Autodesk Inventor part; units mm, degrees
ref_plane "YZ Plane" through (0, 0, 0) normal (1, 0, 0) x (0, 1, 0)
ref_plane "XZ Plane" through (0, 0, 0) normal (0, 1, 0) x (-1, 0, 0)
ref_plane "XY Plane" through (0, 0, 0) normal (0, 0, 1) x (1, 0, 0)
sketch "Sketch1" plane through (0, 0, 0) normal (0, 0, 1) x (1, 0, 0)
  circle A0 centre (0, 0) radius 21
  circle A1 centre (16, 0) radius 2.75
  circle A2 centre (0, 16) radius 2.75
  circle A3 centre (-16, 0) radius 2.75
  circle A4 centre (0, -16) radius 2.75
  circle A5 centre (0, 0) radius 11.1
  dimension "d0" = 42
  dimension "d1" = 5.5
  dimension "d2" = 16
  dimension "d5" = 360
  dimension "d7" = 22.2
extrude "Extrusion1" add sketch "Sketch1" along normal blind 15
sketch "Sketch2" plane through (0, 0, 15) normal (0, 0, 1) x (1, 0, 0)
  circle A0 centre (0, 0) radius 19.1
  dimension "d10" = 38.2
extrude "Extrusion2" cut sketch "Sketch2" against normal blind 2.3
chamfer "Chamfer1" distance 0.5 angle 45 9 edges at (-21, 0, 0) (-21, 0, 15) (-11.1, 0, 0) (-2.75, -16, 0) (-2.75, 16, 0) (13.25, 0, 0) (-18.75, 0, 0) (-11.1, 0, 12.7) (-19.1, 0, 15)
properties part number "spacer nema23" material "PC/ABS Plastic"
The model under review builds one solid part; all positions refer to its coordinate system, in mm. A direction names the side the tool comes from. Round coordinates to 2 decimals unless told otherwise and drop trailing zeros. Loops run counter-clockwise (first coordinate to the right, second up) from the corner with the lowest first, then second, coordinate; pieces in that order, holes last. Notation, with made-up numbers: M 38.25,-10.5 L 77.25,-10.5 A23 ccw 77.25,9.5 Z; hole C 40,-37.5 d3. An arc over 180 degrees is marked long. Answer as a JSON object with one key per item and string values.
Item 1: Clearance check with flat-ended pins moving along their axes: P1, Ø4, axis at y = -13.5, z = 8, coming from the -X side; P2, Ø12, axis at x = 8.5, y = 15, coming from the -Z side; P3, Ø1.5, axis at x = 0.5, y = 11, coming from the +Z side; P4, Ø4, axis at y = -11, z = 12, coming from the -X side. State where each tip first meets the part, or that it passes through.
Check sheet entries:
{"P1": "x = -17.57", "P2": "z = 0", "P3": "z = 12.7", "P4": "x = -18.97"}
Item 2: We need section A-A, the plane y = 0. State how many separate pieces and enclosed holes the cut face has, and give its area (3 significant figures).
Check sheet entries:
{"separate pieces": "4", "enclosed holes": "0", "area": "119 mm2"}
Item 3: For line 1 along Y through (x, z) = (0, 10); line 2 along Y through (x, z) = (2, 11.25); line 3 along Y through (x, z) = (0, 13.95), list the stretches that pass through material, from the lowest coordinate up.
Check sheet entries:
{"line 1": "-21 to -18.75, -13.25 to -11.1, 11.1 to 13.25, 18.75 to 21", "line 2": "-20.9 to -17.89, -14.11 to -10.92, 10.92 to 14.11, 17.89 to 20.9", "line 3": "-21 to -19.1, 19.1 to 21"}
Item 4: The part is to be moulded in two halves that separate along Y. For faces 3 (the face through (11, -17, 15)), 4 (the face through (20.03, -6.31, 7.4)), 5 (the face through (12, 0, 12.7)), say which applies: +Y half, -Y half, draft (parallel to the pull), parting line (faces both ways), or undercut.
Check sheet entries:
{"face 3": "draft", "face 4": "parting line", "face 5": "undercut"}
Item 5: Tool access review of faces 1 (the face through (-15.16, -11.62, 13.61)), 2 (the face through (13.253, -0.121, 6.515)): name each direction out of +Z, -Z, +X, -X, +Y, -Y from which nothing blocks a thin tool from reaching the whole face with its end or side.
Check sheet entries:
{"face 1": "+Z", "face 2": "+Z, -Z"}
Item 6: We need section C-C, the plane z = 13.75. State the section outline as (x, y) points.
Check sheet entries:
{"outline": "C 0,0 d42; hole C 0,0 d38.2"}
Item 7: We need section B-B, the plane z = 3. State the section outline as (x, y) points, and give its area (3 significant figures).
Check sheet entries:
{"outline": "C 0,0 d42; hole C -16,0 d5.5; hole C 0,0 d22.2; hole C 0,-16 d5.5; hole C 0,16 d5.5; hole C 16,0 d5.5", "area": "903 mm2"}
